Work out the finished part from the listing and answer in its coordinate system (mm). Face numbers are marked on the shaded views. Coordinates: 2 decimals unless noted, no trailing zeros. Loops run counter-clockwise (first coordinate to the right, second up) from the corner with the lowest first, then second, coordinate; pieces in that order, holes last. Notation, with made-up numbers: (71.5, 56) - (100.5, 56) arc R19 cw to (100.5, 86) - close; hole circle Ø3 at (25.5, 24). An arc over 180 degrees is marked (long way). Write each question's results on one line, items separated by ' | '. Start each with the question number.
1. Determine the mould class of the marked faces 1 and 2 for opening direction X: released by +X, released by -X, zero draft, split by the parting line, or undercut.
2. A cutting plane is placed at D-D on x = 0. Determine the outline of the cut face in (y, z).
3. Each of these flat-tipped pins is pushed along its axis until it touches: P1, Ø6, axis at x = 3, z = 41.5, coming from the -Y side; P2, Ø1.5, axis at x = 6.5, y = -1.5, coming from the +Z side; P3, Ø1.2, axis at x = 1, z = 0.5, coming from the +Y side. Where does it stop, or does it pass through?
4. A cutting plane is placed at B-B on y = 0. Determine the outline of the cut face in (x, z).
5. A cutting plane is placed at C-C on z = 11.5. Determine the outline of the cut face in (x, y), then the cut area to 3 significant figures.
6. A cutting plane is placed at A-A on x = 6. Determine the outline of the cut face in (y, z), then the cut area to 3 significant figures.
7. Find the intervals of material crossed by line 1 along Z through (x, y) = (-1, -1.75); line 2 along Z through (x, y) = (6, -3); line 3 along Y through (x, z) = (4.25, 42), in increasing order. Write a range as [from, to].
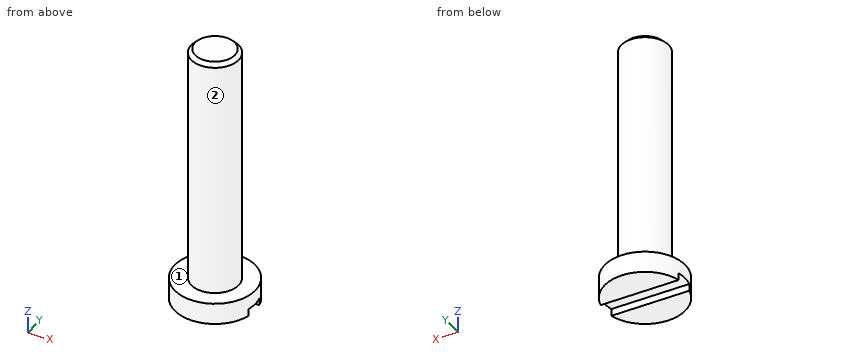
from build123d import *

# Parameters (mm, degrees)
SKETCH_1_R               = 8.5
EXTRUDE_1_DEPTH          = 4.5
SKETCH_2_R               = 5
EXTRUDE_2_DEPTH          = 55.5
CUT_EXTRUDE_1_DEPTH      = 57.786882288
CUT_EXTRUDE_1_DEPTH_BACK = 1.5
SKETCH_5_W               = 17
SKETCH_5_H               = 4


# Read off the part's stored shape, not the designer's step: M10 机械螺纹 螺柱1
with BuildPart() as part:
    # 草图1 → 凸台-拉伸1 (new body)
    with BuildSketch(Plane.XY):
        Circle(SKETCH_1_R)
    extrude(amount=EXTRUDE_1_DEPTH)

    # 草图2 → 凸台-拉伸2 (add)
    with BuildSketch(Plane.XY):
        Circle(SKETCH_2_R)
    extrude(amount=EXTRUDE_2_DEPTH)

    # M10 机械螺纹 螺柱1 outline → M10 机械螺纹 螺柱1 (revolve, cut)
    with BuildSketch(Plane.XZ):
        Polygon((5, 55.5), (4.188, 55.5), (5, 54.688), align=None)
    revolve(axis=Axis((0, 0, 0), (0, 0, 1)), mode=Mode.SUBTRACT)

    # 草图5 → 切除-拉伸-薄壁1 (cut, two sides: drawn at the far end of the back side and taken through both)
    with BuildSketch(Plane(origin=(0, 0, 0), x_dir=(-1, 0, 0), z_dir=(0, 0, -1)).offset(-CUT_EXTRUDE_1_DEPTH_BACK)):
        Rectangle(SKETCH_5_W, SKETCH_5_H)
    extrude(amount=CUT_EXTRUDE_1_DEPTH + CUT_EXTRUDE_1_DEPTH_BACK, mode=Mode.SUBTRACT)


solid = part.part
Values:
1) face 1: zero draft | face 2: split by the parting line
2) outline: (-8.5, 0) - (-2, 0) - (-2, 1.5) - (2, 1.5) - (2, 0) - (8.5, 0) - (8.5, 4.5) - (5, 4.5) - (5, 54.69) - (4.19, 55.5) - (-4.19, 55.5) - (-5, 54.69) - (-5, 4.5) - (-8.5, 4.5) - close
3) P1: y = -5 | P2: z = 4.5 | P3: y = 8.49
4) outline: (-8.5, 1.5) - (8.5, 1.5) - (8.5, 4.5) - (5, 4.5) - (5, 54.69) - (4.19, 55.5) - (-4.19, 55.5) - (-5, 54.69) - (-5, 4.5) - (-8.5, 4.5) - close
5) outline: circle Ø10 at (0, 0) | area: 78.5 mm^2
6) outline: (-6.02, 0) - (-2, 0) - (-2, 1.5) - (2, 1.5) - (2, 0) - (6.02, 0) - (6.02, 4.5) - (-6.02, 4.5) - close | area: 48.2 mm^2
7) line 1: [1.5, 55.5] | line 2: [0, 4.5] | line 3: [-2.63, 2.63]
